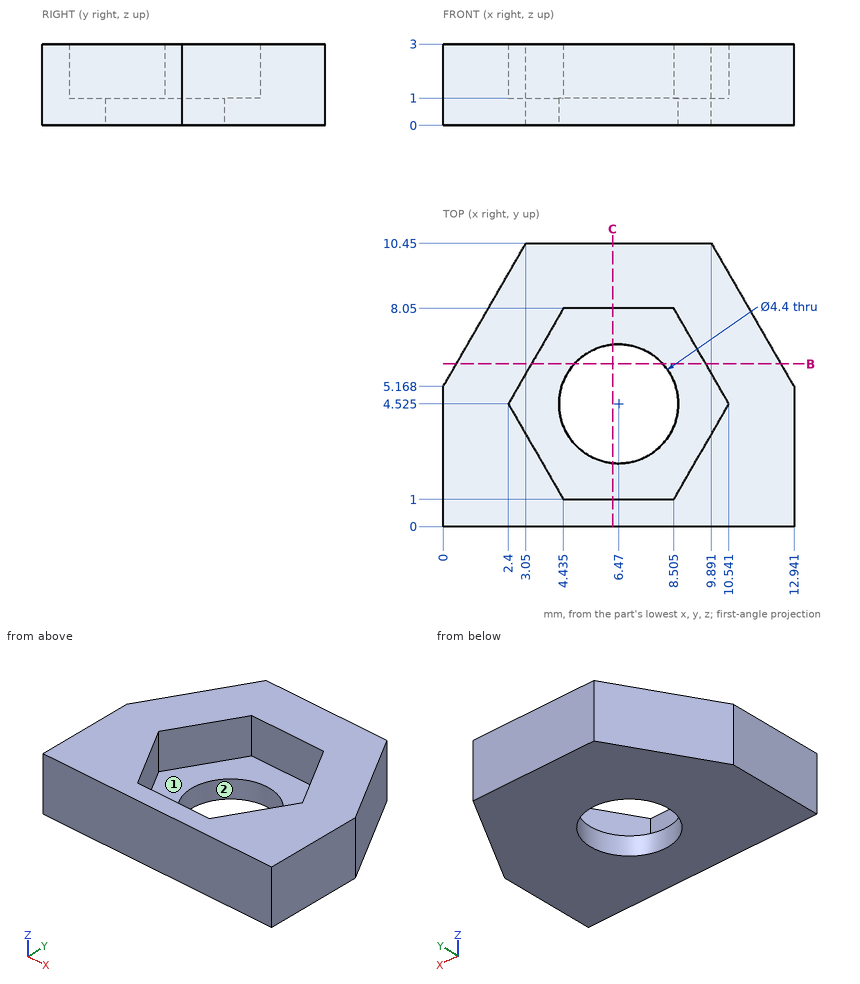
Drawing for the job (mm, zero at the part's lowest x, y, z). A direction names the side the tool comes from. Round coordinates to 2 decimals unless told otherwise and drop trailing zeros. Write each loop counter-clockwise with the first axis right and the second up, starting at its lowest first coordinate (ties: lowest second). Pieces come first, ordered by that corner, then holes. Notation, with made-up numbers: M -38,86 L -2,86 A25 ccw -2,111 Z; hole C 15.25,12.5 d11. An arc over 180 degrees is marked long. Answer in a Markdown table with one row per item.
1. Saw through at C-C (x = 6.25). List the corners of the cut face in (y, z).
Geometry check:
| item | result |
|---|---|
| outline | M 0,0 L 2.34,0 L 2.34,1 L 1,1 L 1,3 L 0,3 Z; M 6.71,0 L 10.45,0 L 10.45,3 L 8.05,3 L 8.05,1 L 6.71,1 Z |
2. Probe L1, parallel to Y at x = 7.5, z = 1.95; L2, parallel to X at y = 5, z = 0.35; L3, parallel to X at y = 4, z = 2.7 (1 decimal). List the from-to ranges inside material, lowest first. Write a range as [from, to].
Geometry check:
| item | result |
|---|---|
| L1 | [0, 1], [8.05, 10.45] |
| L2 | [0, 4.32], [8.62, 12.94] |
| L3 | [0, 2.7], [10.2, 12.9] |
3. Saw through at B-B (y = 6). List the corners of the cut face in (x, z), and give its area (3 significant figures).
Geometry check:
| item | result |
|---|---|
| outline | M 0.48,0 L 4.84,0 L 4.84,1 L 3.25,1 L 3.25,3 L 0.48,3 Z; M 8.1,0 L 12.46,0 L 12.46,3 L 9.69,3 L 9.69,1 L 8.1,1 Z |
| area | 19.8 mm2 |
4. Which spindle directions (+Z, -Z, +X, -X, +Y, -Y) get a long thin tool onto all of the face, cutting with end or side? Do the marked faces 1 and 2. Say none if no direction does.
Geometry check:
| item | result |
|---|---|
| face 1 | +Z |
| face 2 | +Z, -Z |
5. Flat gauge pin, fed straight in: P1, Ø1, axis at y = 6, z = 1.5, coming from the -X side. Where does the tip first touch, or does it go through?
Geometry check:
| item | result |
|---|---|
| P1 | x = 0.19 |
